from build123d import *

# Parameters (mm, degrees)
SKETCH1_R           = 12.5
SKETCH1_R_2         = 7.5
BOSS_EXTRUDE1_DEPTH = 2
SKETCH1_3_R         = 7.5
SKETCH1_3_R_2       = 5
BOSS_EXTRUDE2_DEPTH = 8
CUT_EXTRUDE1_DEPTH  = 2
SKETCH3_R           = 1.25
CUT_EXTRUDE2_DEPTH  = 2


with BuildPart() as part:
    # Sketch1 → Boss-Extrude1 (new body)
    with BuildSketch(Plane(origin=(0, 0, 0), x_dir=(1, 0, 0), z_dir=(0, 1, 0))):
        with Locations(Location((0, 0, 0), (0, 0, 270))):
            Circle(SKETCH1_R)
        with Locations(Location((0, 0, 0), (0, 0, 270))):
            Circle(SKETCH1_R_2, mode=Mode.SUBTRACT)
    extrude(amount=BOSS_EXTRUDE1_DEPTH)

    # Sketch1<3> → Boss-Extrude2 (add)
    with BuildSketch(Plane(origin=(0, 0, 0), x_dir=(1, 0, 0), z_dir=(0, 1, 0))):
        with Locations(Location((0, 0, 0), (0, 0, 270))):
            Circle(SKETCH1_3_R)
        with Locations(Location((0, 0, 0), (0, 0, 270))):
            Circle(SKETCH1_3_R_2, mode=Mode.SUBTRACT)
    extrude(amount=BOSS_EXTRUDE2_DEPTH)

    # Sketch2 → Cut-Extrude1 (cut)
    with BuildSketch(Plane(origin=(0, 2, 0), x_dir=(1, 0, 0), z_dir=(0, 1, 0))):
        with BuildLine():
            Line((-4.25, -13.5), (4.25, -13.5))
            Line((4.25, -13.5), (4.25, -9.5))
            ThreePointArc((4.25, -9.5), (3.957106781, -8.792893219), (3.25, -8.5))
            Line((3.25, -8.5), (-3.25, -8.5))
            ThreePointArc((-3.25, -8.5), (-3.957106781, -8.792893219), (-4.25, -9.5))
            Line((-4.25, -9.5), (-4.25, -13.5))
        make_face()
    extrude(amount=-CUT_EXTRUDE1_DEPTH, mode=Mode.SUBTRACT)

    # Sketch3 → Cut-Extrude2 (cut)
    with BuildSketch(Plane(origin=(0, 2, 0), x_dir=(1, 0, 0), z_dir=(0, 1, 0))):
        with Locations(Location((0, 10.25, 0), (0, 0, 270))):
            Circle(SKETCH3_R)
        with Locations(Location((8.876760389, -5.125, 0), (0, 0, 270))):
            Circle(SKETCH3_R)
        with Locations(Location((-8.876760389, -5.125, 0), (0, 0, 270))):
            Circle(SKETCH3_R)
    extrude(amount=-CUT_EXTRUDE2_DEPTH, mode=Mode.SUBTRACT)


solid = part.part
Could you check a few things on this model? Use its own coordinates, in mm. A direction names the side the tool comes from. Give positions to 0.01 mm unless a question says otherwise; leave off trailing zeros. Order: outer loops, then holes, each group sorted by start corner. A loop starts at its lowest first (then second) coordinate and runs counter-clockwise, first axis right, second up.
Item 1: I'm going to push flat-ended pins straight in: pin 1 (3 mm diameter, centred on x = 8.88, z = 5.12, fed in from +Y); pin 2 (1.6 mm diameter, centred on y = 1, z = 10, fed in from +X); pin 3 (2 mm diameter, centred on x = 1, y = 1, fed in from +Z); pin 4 (12 mm diameter, centred on x = 3.5, z = -1, fed in from +Y). Where does each tip first touch, or does it pass through?
Item 2: I need wall thicknesses on line 1 (X direction, y = 4.25, z = 0); line 2 (Y direction, x = -7.75, z = 3.75); line 3 (Z direction, x = 4.5, y = 5.25). Which ranges of each line are inside material? Lowest first, please.
Item 3: If we section it at C-C, the plane z = 6: Write out the boundary of the cut face in (x, y).
Item 4: If we section it at B-B, the plane x = 0: Write out the boundary of the cut face in (y, z), plus the area to 3 significant figures.
Item 5: If we section it at A-A, the plane z = 10: Write out the boundary of the cut face in (x, y).
Item 6: If we section it at D-D, the plane x = -8: Write out the boundary of the cut face in (y, z), plus the area to 3 significant figures.
Item 7: If we mould it in two halves opening along Z, with no side actions, what happens to faces 4 (the face through (-10.097, 1.014, 4.854)), 5 (the face through (-4.88, 3.94, -1.08)), 6 (the face through (0.49, 0.99, -12.49)), 7 (the face through (4.25, 1, 11))? For each: pulls with the +Z half, pulls with the -Z half, needs draft (parallel to the pull), parting line crosses it, or undercut.
Item 8: For faces 1 (the face through (-5, 2, -6)), 2 (the face through (-5, 8, 2)), 3 (the face through (-3.949, 1.014, 8.785)), which set-ups out of +Z, -Z, +X, -X, +Y, -Y let a thin tool reach every point of the face, with its end or its side?
Values:
1. pin 1: stops at y = 2
1. pin 2: stops at x = 8.46
1. pin 3: stops at z = 8.5
1. pin 4: stops at y = 8
2. line 1: x = -7.5 to -5, 5 to 7.5
2. line 2: y = 0 to 2
2. line 3: z = -6 to -2.18, 2.18 to 6
3. outline: (-10.97, 0) - (-9.77, 0) - (-9.77, 2) - (-10.97, 2) - close; (-7.98, 0) - (7.98, 0) - (7.98, 2) - (4.5, 2) - (4.5, 8) - (-4.5, 8) - (-4.5, 2) - (-7.98, 2) - close; (9.77, 0) - (10.97, 0) - (10.97, 2) - (9.77, 2) - close
4. outline: (0, -12.5) - (2, -12.5) - (2, -11.5) - (0, -11.5) - close; (0, -9) - (2, -9) - (2, -7.5) - (8, -7.5) - (8, -5) - (0, -5) - close; (0, 5) - (8, 5) - (8, 7.5) - (2, 7.5) - (2, 8.5) - (0, 8.5) - close
4. area: 47.0 mm2
5. outline: (-7.5, 0) - (-4.25, 0) - (-4.25, 2) - (-7.5, 2) - close; (4.25, 0) - (7.5, 0) - (7.5, 2) - (4.25, 2) - close
6. outline: (0, -9.6) - (2, -9.6) - (2, 4.23) - (0, 4.23) - close; (0, 6.02) - (2, 6.02) - (2, 9.6) - (0, 9.6) - close
6. area: 34.9 mm2
7. face 4: undercut
7. face 5: undercut
7. face 6: parting line crosses it
7. face 7: needs draft
8. face 1: +Y
8. face 2: +Z, -Z, +X, -X, +Y
8. face 3: +Z, +Y, -Y
